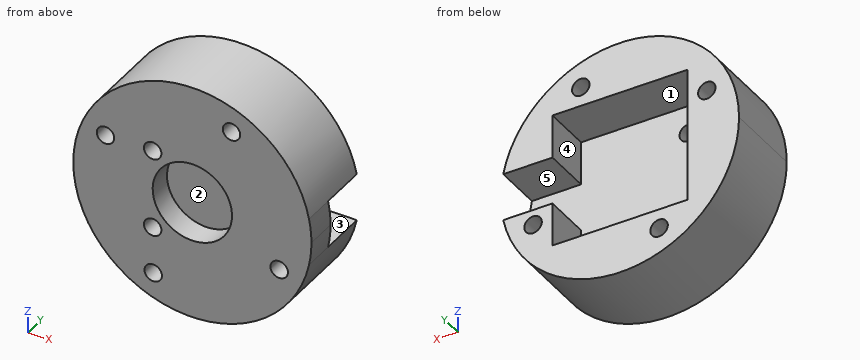
from build123d import *

# Parameters (mm, degrees)
SKETCH1_R                   = 1.1
BOSS_EXTRUDE1_DEPTH         = 10
ACCEL_START                 = 4
ACCEL_CUTOUT_DEPTH          = 6
SKETCH1_4_R                 = 1.1
ACCEL_MOUNT_HOLES_DEPTH     = 24.452078799
SKETCH2_R                   = 5
REAR_THREAD_INSERT_DEPTH    = 3
SKETCH1_5_R                 = 1.1
LAYERSCREW_HOLES_DEPTH      = 24.452078799
LAYERSCREW_HOLES_MORE_COUNT = 4


with BuildPart() as part:
    # Sketch1 → Boss-Extrude1 (new body)
    # profile 1 of 17: a face of its own
    with BuildSketch(Plane(origin=(0, 0, 0), x_dir=(1, 0, 0), z_dir=(0, 1, 0))):
        with BuildLine():
            ThreePointArc((14.696938457, 3), (-1.50763443, 14.924042295), (-15, 0))
            Line((-15, 0), (-8.5, 0))
            Line((-8.5, 0), (-8.5, 8.5))
            Line((-8.5, 8.5), (8.5, 8.5))
            Line((8.5, 8.5), (8.5, 3))
            Line((8.5, 3), (14.696938457, 3))
        make_face()
        with Locations((10.940488944, 4.930081304)):
            Circle(SKETCH1_R, mode=Mode.SUBTRACT)
    # profile 2 of 17: a face of its own
    with BuildSketch(Plane(origin=(0, 0, 0), x_dir=(1, 0, 0), z_dir=(0, 1, 0))):
        with BuildLine():
            Line((-8.5, 0), (-15, 0))
            ThreePointArc((-15, 0), (-1.50763443, -14.924042295), (14.696938457, -3))
            Line((14.696938457, -3), (8.5, -3))
            Line((8.5, -3), (8.5, -8.5))
            Line((8.5, -8.5), (-8.5, -8.5))
            Line((-8.5, -8.5), (-8.5, 0))
        make_face()
    # profile 3 of 17: a face of its own
    with BuildSketch(Plane(origin=(0, 0, 0), x_dir=(1, 0, 0), z_dir=(0, 1, 0))):
        with BuildLine():
            Line((8.5, -3), (14.696938457, -3))
            ThreePointArc((14.696938457, -3), (14.924042295, -1.50763443), (15, 0))
            Line((15, 0), (8.5, 0))
            Line((8.5, 0), (8.5, -3))
        make_face()
    # profile 4 of 17: a face of its own
    with BuildSketch(Plane(origin=(0, 0, 0), x_dir=(1, 0, 0), z_dir=(0, 1, 0))):
        with BuildLine():
            ThreePointArc((15, 0), (14.924042295, 1.50763443), (14.696938457, 3))
            Line((14.696938457, 3), (8.5, 3))
            Line((8.5, 3), (8.5, 0))
            Line((8.5, 0), (15, 0))
        make_face()
    # profile 5 of 17: a face of its own
    with BuildSketch(Plane(origin=(0, 0, 0), x_dir=(1, 0, 0), z_dir=(0, 1, 0))):
        with BuildLine():
            Line((-8.5, 8.5), (-8.5, 0))
            Line((-8.5, 0), (-5, 0))
            Line((-5, 0), (-5, 3.9))
            ThreePointArc((-5, 3.9), (-5.777817459, 5.777817459), (-3.9, 5))
            Line((-3.9, 5), (5, 5))
            Line((5, 5), (5, 0))
            Line((5, 0), (8.5, 0))
            Line((8.5, 0), (8.5, 3))
            Line((8.5, 3), (8.5, 8.5))
            Line((8.5, 8.5), (-8.5, 8.5))
        make_face()
    # profile 6 of 17: a face of its own
    with BuildSketch(Plane(origin=(0, 0, 0), x_dir=(1, 0, 0), z_dir=(0, 1, 0))):
        with BuildLine():
            ThreePointArc((-3.9, 5), (-5.777817459, 5.777817459), (-5, 3.9))
            Line((-5, 3.9), (-5, 5))
            Line((-5, 5), (-3.9, 5))
        make_face()
    # profile 7 of 17: a face of its own
    with BuildSketch(Plane(origin=(0, 0, 0), x_dir=(1, 0, 0), z_dir=(0, 1, 0))):
        with BuildLine():
            Line((-5, 5), (-5, 3.9))
            ThreePointArc((-5, 3.9), (-4.222182541, 4.222182541), (-3.9, 5))
            Line((-3.9, 5), (-5, 5))
        make_face()
    # profile 8 of 17: a face of its own
    with BuildSketch(Plane(origin=(0, 0, 0), x_dir=(1, 0, 0), z_dir=(0, 1, 0))):
        with BuildLine():
            Line((-5, 3.9), (-5, 0))
            Line((-5, 0), (5, 0))
            Line((5, 0), (5, 5))
            Line((5, 5), (-3.9, 5))
            ThreePointArc((-3.9, 5), (-4.222182541, 4.222182541), (-5, 3.9))
        make_face()
    # profile 9 of 17: a face of its own
    with BuildSketch(Plane(origin=(0, 0, 0), x_dir=(1, 0, 0), z_dir=(0, 1, 0))):
        with BuildLine():
            ThreePointArc((-3.9, 5), (-5.777817459, 5.777817459), (-5, 3.9))
            Line((-5, 3.9), (-5, 5))
            Line((-5, 5), (-3.9, 5))
        make_face()
    # profile 10 of 17: a face of its own
    with BuildSketch(Plane(origin=(0, 0, 0), x_dir=(1, 0, 0), z_dir=(0, 1, 0))):
        with BuildLine():
            Line((-5, 5), (-5, 3.9))
            ThreePointArc((-5, 3.9), (-4.222182541, 4.222182541), (-3.9, 5))
            Line((-3.9, 5), (-5, 5))
        make_face()
    # profile 11 of 17: a face of its own
    with BuildSketch(Plane(origin=(0, 0, 0), x_dir=(1, 0, 0), z_dir=(0, 1, 0))):
        with BuildLine():
            Line((-5, 0), (-8.5, 0))
            Line((-8.5, 0), (-8.5, -8.5))
            Line((-8.5, -8.5), (8.5, -8.5))
            Line((8.5, -8.5), (8.5, -3))
            Line((8.5, -3), (8.5, 0))
            Line((8.5, 0), (5, 0))
            Line((5, 0), (5, -5))
            Line((5, -5), (-3.9, -5))
            ThreePointArc((-3.9, -5), (-5.777817459, -5.777817459), (-5, -3.9))
            Line((-5, -3.9), (-5, 0))
        make_face()
    # profile 12 of 17: a face of its own
    with BuildSketch(Plane(origin=(0, 0, 0), x_dir=(1, 0, 0), z_dir=(0, 1, 0))):
        with BuildLine():
            ThreePointArc((-3.9, -5), (-4.222182541, -4.222182541), (-5, -3.9))
            Line((-5, -3.9), (-5, -5))
            Line((-5, -5), (-3.9, -5))
        make_face()
    # profile 13 of 17: a face of its own
    with BuildSketch(Plane(origin=(0, 0, 0), x_dir=(1, 0, 0), z_dir=(0, 1, 0))):
        with BuildLine():
            Line((-5, -5), (-5, -3.9))
            ThreePointArc((-5, -3.9), (-5.777817459, -5.777817459), (-3.9, -5))
            Line((-3.9, -5), (-5, -5))
        make_face()
    # profile 14 of 17: a face of its own
    with BuildSketch(Plane(origin=(0, 0, 0), x_dir=(1, 0, 0), z_dir=(0, 1, 0))):
        with BuildLine():
            ThreePointArc((-3.9, -5), (-4.222182541, -4.222182541), (-5, -3.9))
            Line((-5, -3.9), (-5, -5))
            Line((-5, -5), (-3.9, -5))
        make_face()
    # profile 15 of 17: a face of its own
    with BuildSketch(Plane(origin=(0, 0, 0), x_dir=(1, 0, 0), z_dir=(0, 1, 0))):
        with BuildLine():
            Line((-5, -5), (-5, -3.9))
            ThreePointArc((-5, -3.9), (-5.777817459, -5.777817459), (-3.9, -5))
            Line((-3.9, -5), (-5, -5))
        make_face()
    # profile 16 of 17: a face of its own
    with BuildSketch(Plane(origin=(0, 0, 0), x_dir=(1, 0, 0), z_dir=(0, 1, 0))):
        with BuildLine():
            Line((5, 0), (-5, 0))
            Line((-5, 0), (-5, -3.9))
            ThreePointArc((-5, -3.9), (-4.222182541, -4.222182541), (-3.9, -5))
            Line((-3.9, -5), (5, -5))
            Line((5, -5), (5, 0))
        make_face()
    # profile 17 of 17: a face of its own
    with BuildSketch(Plane(origin=(0, 0, 0), x_dir=(1, 0, 0), z_dir=(0, 1, 0))):
        with Locations((10.940488944, 4.930081304)):
            Circle(SKETCH1_R)
    extrude(amount=BOSS_EXTRUDE1_DEPTH)

    # Sketch1_3 → accel cutout (cut)
    with BuildSketch(Plane(origin=(0, 0, 0), x_dir=(1, 0, 0), z_dir=(0, 1, 0)).offset(ACCEL_START)):
        with BuildLine():
            Line((-8.5, 8.5), (-8.5, 0))
            Line((-8.5, 0), (-5, 0))
            Line((-5, 0), (-5, 3.9))
            ThreePointArc((-5, 3.9), (-5.777817459, 5.777817459), (-3.9, 5))
            Line((-3.9, 5), (5, 5))
            Line((5, 5), (5, 0))
            Line((5, 0), (8.5, 0))
            Line((8.5, 0), (8.5, 3))
            Line((8.5, 3), (8.5, 8.5))
            Line((8.5, 8.5), (-8.5, 8.5))
        make_face()
        with BuildLine():
            Line((-5, 3.9), (-5, 0))
            Line((-5, 0), (5, 0))
            Line((5, 0), (5, 5))
            Line((5, 5), (-3.9, 5))
            ThreePointArc((-3.9, 5), (-4.222182541, 4.222182541), (-5, 3.9))
        make_face()
        with BuildLine():
            Line((5, 0), (-5, 0))
            Line((-5, 0), (-5, -3.9))
            ThreePointArc((-5, -3.9), (-4.222182541, -4.222182541), (-3.9, -5))
            Line((-3.9, -5), (5, -5))
            Line((5, -5), (5, 0))
        make_face()
        with BuildLine():
            Line((-5, 0), (-8.5, 0))
            Line((-8.5, 0), (-8.5, -8.5))
            Line((-8.5, -8.5), (8.5, -8.5))
            Line((8.5, -8.5), (8.5, -3))
            Line((8.5, -3), (8.5, 0))
            Line((8.5, 0), (5, 0))
            Line((5, 0), (5, -5))
            Line((5, -5), (-3.9, -5))
            ThreePointArc((-3.9, -5), (-5.777817459, -5.777817459), (-5, -3.9))
            Line((-5, -3.9), (-5, 0))
        make_face()
        with BuildLine():
            ThreePointArc((15, 0), (14.924042295, 1.50763443), (14.696938457, 3))
            Line((14.696938457, 3), (8.5, 3))
            Line((8.5, 3), (8.5, 0))
            Line((8.5, 0), (15, 0))
        make_face()
        with BuildLine():
            Line((8.5, -3), (14.696938457, -3))
            ThreePointArc((14.696938457, -3), (14.924042295, -1.50763443), (15, 0))
            Line((15, 0), (8.5, 0))
            Line((8.5, 0), (8.5, -3))
        make_face()
    extrude(amount=ACCEL_CUTOUT_DEPTH, mode=Mode.SUBTRACT)

    # Sketch1_4 → accel mount holes (cut, through all)
    with BuildSketch(Plane(origin=(0, 0, 0), x_dir=(1, 0, 0), z_dir=(0, 1, 0))):
        with Locations(Location((-5, 5, 0), (0, 0, 270))):
            Circle(SKETCH1_4_R)
        with Locations(Location((-5, -5, 0), (0, 0, 270))):
            Circle(SKETCH1_4_R)
    extrude(amount=ACCEL_MOUNT_HOLES_DEPTH, mode=Mode.SUBTRACT)

    # Sketch2 → rear thread insert (cut)
    with BuildSketch(Plane(origin=(0, 0, 0), x_dir=(1, 0, 0), z_dir=(0, 1, 0))):
        with Locations(Location((0, 0, 0), (0, 0, 270))):
            Circle(SKETCH2_R)
    extrude(amount=REAR_THREAD_INSERT_DEPTH, mode=Mode.SUBTRACT)

    # Sketch1_5 → layerscrew holes (cut, through all)
    with BuildSketch(Plane(origin=(0, 0, 0), x_dir=(1, 0, 0), z_dir=(0, 1, 0))):
        with Locations(Location((10.940488944, 4.930081304, 0), (0, 0, 270))):
            Circle(SKETCH1_5_R)
    layerscrew_holes = extrude(amount=LAYERSCREW_HOLES_DEPTH, mode=Mode.SUBTRACT)

    # layerscrew holes more: layerscrew holes ×4 about axis
    layerscrew_holes_more_axis = Axis((0, 0, 0), (0, 1, 0))
    for i in range(1, LAYERSCREW_HOLES_MORE_COUNT):
        add(layerscrew_holes.rotate(layerscrew_holes_more_axis, i * 360 / LAYERSCREW_HOLES_MORE_COUNT), mode=Mode.SUBTRACT)


solid = part.part
For this review, take the finished solid that the model builds, in its own axes (mm). Face numbers are marked on the shaded views. A direction names the side the tool comes from. Give positions to 0.01 mm unless a question says otherwise; leave off trailing zeros. Order: outer loops, then holes, each group sorted by start corner. A loop starts at its lowest first (then second) coordinate and runs counter-clockwise, first axis right, second up. Notation, with made-up numbers: (36, 10) -> (40, 10) arc R29 cw to (40, 43) -> close; hole circle Ø6 at (36, 68.25). An arc over 180 degrees is marked (long way). Write item = value, one per line.
1) We need section B-B, the plane y = 5. Give the boundary of the cut face in (x, z), and give its area (3 significant figures).
Findings:
outline = (-8.5, -8.5) -> (-8.5, 8.5) -> (8.5, 8.5) -> (8.5, 3) -> (14.7, 3) arc R15 ccw (long way) to (14.7, -3) -> (8.5, -3) -> (8.5, -8.5) -> close; hole circle Ø2.2 at (-10.94, 4.93); hole circle Ø2.2 at (-4.93, -10.94); hole circle Ø2.2 at (4.93, 10.94); hole circle Ø2.2 at (10.94, -4.93)
area = 364 mm^2
2) Draft analysis for pull direction X (two halves, no side actions). For the marked faces 4 and 5, state which applies: pulls with the +X half, pulls with the -X half, needs draft (parallel to the pull), parting line crosses it, or undercut.
Findings:
face_4 = undercut
face_5 = needs draft
3) We need section C-C, the plane z = 7.75. Give the boundary of the cut face in (x, y), and give its area (3 significant figures).
Findings:
outline = (-12.84, 0) -> (12.84, 0) -> (12.84, 10) -> (8.5, 10) -> (8.5, 4) -> (-8.5, 4) -> (-8.5, 10) -> (-12.84, 10) -> close
area = 155 mm^2
4) We need section D-D, the plane y = 1. Give the boundary of the cut face in (x, z).
Findings:
outline = circle Ø30 at (0, 0); hole circle Ø2.2 at (-10.94, 4.93); hole circle Ø2.2 at (-5, -5); hole circle Ø2.2 at (-5, 5); hole circle Ø2.2 at (-4.93, -10.94); hole circle Ø10 at (0, 0); hole circle Ø2.2 at (4.93, 10.94); hole circle Ø2.2 at (10.94, -4.93)
5) To check wall thickness, follow L1, parallel to Z at x = 10, y = 6.75; L2, parallel to X at y = 8, z = -5.5; L3, parallel to Y at x = 10.75, z = 1. State the ranges of each line that lie inside material, in increasing order. Write a range as from..to.
Findings:
L1 = -11.18..-5.5, -4.36..-3, 3..11.18
L2 = -13.96..-8.5, 8.5..10, 11.88..13.96
L3 = 0..4
6) We need section A-A, the plane x = 0. Give the boundary of the cut face in (y, z), and give its area (3 significant figures).
Findings:
outline = (0, -15) -> (10, -15) -> (10, -8.5) -> (4, -8.5) -> (4, 8.5) -> (10, 8.5) -> (10, 15) -> (0, 15) -> (0, 5) -> (3, 5) -> (3, -5) -> (0, -5) -> close
area = 168 mm^2
7) For the marked faces 1, 2 and 3, list the 3-axis set-ups (+Z, -Z, +X, -X, +Y, -Y) from which the entire face can be reached by the end or side of a thin tool; tool diameter is ignored.
Findings:
face_1 = +Y
face_2 = -Y
face_3 = +X, +Y
8) Insertion check: pin 1 (1 mm diameter, centred on x = 11, y = 4.5, fed in from +Z); pin 2 (1.8 mm diameter, centred on x = 11, y = 8.5, fed in from +Z); pin 3 (1.6 mm diameter, centred on y = 7, z = 6, fed in from -X). Each pin has a flat end and moves straight along its axis. Give the tip position at first contact, or say it passes through.
Findings:
pin_1 = 10.71
pin_2 = 11.09
pin_3 = -14.07
